from build123d import *

# Parameters (mm, degrees)
F0_R     = 33
F1_DEPTH = 25
F2_SIZE  = 10
F3_T     = -1.6


with BuildPart() as f1:
    # F0 (on Top) → F1 (new body)
    with BuildSketch(Plane.XY):
        Circle(F0_R)
    extrude(amount=F1_DEPTH)

    # F2
    f2_edges = [f1.edges().sort_by_distance(p)[0] for p in [
        (-33, 0, 0),
    ]]
    chamfer(f2_edges, length=F2_SIZE)

    # F3
    f3_openings = [f1.faces().sort_by_distance(p)[0] for p in [
        (0, 0, 25),
    ]]
    offset(amount=F3_T, openings=f3_openings)


solid = f1.part
Geometry check sheet. Reference: the model listing, model coordinates, mm. A direction names the side the tool comes from. Give positions to 0.01 mm unless a question says otherwise; leave off trailing zeros. Loops run counter-clockwise (first coordinate to the right, second up) from the corner with the lowest first, then second, coordinate; pieces in that order, holes last.
(1) Release check for a two-part mould opening along X. For faces 1 (the flat face through (29.2, -12.1, 25)), 2 (the cylindrical face through (30.5, -12.6, 17.4)), 3 (the conical face through (-18.075, -13.86, 2.04)) record: released by +X, released by -X, zero draft, split by the parting line, or undercut.
From the geometry:
face 1: zero draft
face 2: split by the parting line
face 3: undercut
(2) Section check C-C on z = 21.75. Record the cut outline in (x, y).
From the geometry:
outline: circle Ø66 at (0, 0); hole circle Ø62.8 at (0, 0)
(3) Set-up check for faces 4 (the cylindrical face through (-23.143, 21.222, 17.731)), 5 (the flat face through (0, 0, 0)): record each of +Z, -Z, +X, -X, +Y, -Y from which the full face is reachable in a straight line by a thin tool's end or side.
From the geometry:
face 4: +Z
face 5: -Z, +X, -X, +Y, -Y
(4) Thickness scan on L1, parallel to Y at x = 0, z = 18.25; L2, parallel to Z at x = -16, y = 1; L3, parallel to Y at x = -16, z = 14. Record the ranges inside material, lowest first.
From the geometry:
L1: y = -33 to -31.4, 31.4 to 33
L2: z = 0 to 1.6
L3: y = -28.86 to -27.02, 27.02 to 28.86
(5) Section check A-A on x = 0. Record the cut outline in (y, z).
From the geometry:
outline: (-33, 10) - (-23, 0) - (23, 0) - (33, 10) - (33, 25) - (31.4, 25) - (31.4, 10.66) - (22.34, 1.6) - (-22.34, 1.6) - (-31.4, 10.66) - (-31.4, 25) - (-33, 25) - close
(6) Depth check by flat-ended pin: pin 1 Ø12 at (y, z) = (12.5, 10.5) entering from -X; pin 2 Ø8 at (y, z) = (11.5, 13) entering from -X; pin 3 Ø5 at (x, z) = (-6.5, 3.5) entering from +Y; pin 4 Ø5 at (x, y) = (6, -20) entering from -Z. Enter the tip coordinate at first touch or a pass-through.
From the geometry:
pin 1: stops at x = -32.35
pin 2: stops at x = -32.14
pin 3: stops at y = 28.32
pin 4: stops at z = 0
